Work out the finished part from the listing and answer in its coordinate system (mm). A direction names the side the tool comes from. Round coordinates to 2 decimals unless told otherwise and drop trailing zeros. Order: outer loops, then holes, each group sorted by start corner. A loop starts at its lowest first (then second) coordinate and runs counter-clockwise, first axis right, second up. Notation, with made-up numbers: M 43,63.5 L 63,63.5 A27 cw 63,100.5 Z; hole C 3,3 d3. An arc over 180 degrees is marked long. Return JSON: item names as keys, results as strings.
from build123d import *

# Parameters (mm, degrees)
SKETCH013_W   = 18.2
SKETCH013_H   = 20.2
SKETCH013_W_2 = 7.8
SKETCH013_H_2 = 4.8
PAD013_DEPTH  = 5


with BuildPart() as part:
    # Sketch013 → Pad013 (new body)
    with BuildSketch(Plane(origin=(0, -2.5, 80), x_dir=(1, 0, 0), z_dir=(0, 0, 1))):
        Rectangle(SKETCH013_W, SKETCH013_H)
        with Locations((0, 5)):
            Rectangle(SKETCH013_W_2, SKETCH013_H_2, mode=Mode.SUBTRACT)
        with Locations((0, -5)):
            Rectangle(SKETCH013_W_2, SKETCH013_H_2, mode=Mode.SUBTRACT)
    extrude(amount=PAD013_DEPTH)


solid = part.part
Item 1: Find section B-B (z = 83.45). Determine the outline of the cut face in (x, y).
Output:
{"outline": "M -9.1,-12.6 L 9.1,-12.6 L 9.1,7.6 L -9.1,7.6 Z; hole M -3.9,-9.9 L 3.9,-9.9 L 3.9,-5.1 L -3.9,-5.1 Z; hole M -3.9,0.1 L 3.9,0.1 L 3.9,4.9 L -3.9,4.9 Z"}
Item 2: Find section C-C (x = 1). Determine the outline of the cut face in (y, z).
Output:
{"outline": "M -12.6,80 L -9.9,80 L -9.9,85 L -12.6,85 Z; M -5.1,80 L 0.1,80 L 0.1,85 L -5.1,85 Z; M 4.9,80 L 7.6,80 L 7.6,85 L 4.9,85 Z"}
Item 3: The mould has two halves that part along Y. Classify faces 3 (the flat face through (0, 4.9, 82)), 4 (the flat face through (0, -2, 80)), 5 (the flat face through (0, -12.6, 82)): pulls with the +Y half, pulls with the -Y half, needs draft (parallel to the pull), parting line crosses it, or undercut.
Output:
{"face 3": "undercut", "face 4": "needs draft", "face 5": "pulls with the -Y half"}
Item 4: Consider line 1 along Y through (x, z) = (-3, 83.7); line 2 along X through (y, z) = (0.75, 80.6). Determine where each line is inside the solid, lowest interval first. Write a range as [from, to].
Output:
{"line 1": "y = [-12.6, -9.9], [-5.1, 0.1], [4.9, 7.6]", "line 2": "x = [-9.1, -3.9], [3.9, 9.1]"}
Item 5: Which of the six approach directions +Z, -Z, +X, -X, +Y, -Y give full straight-line access (tool end or side, diameter ignored) to faces 1 (the flat face through (3.9, -8, 82)), 2 (the flat face through (0, -2, 85))?
Output:
{"face 1": "+Z, -Z", "face 2": "+Z, +X, -X, +Y, -Y"}
Item 6: Find section A-A (y = -8.5). Determine the outline of the cut face in (x, z).
Output:
{"outline": "M -9.1,80 L -3.9,80 L -3.9,85 L -9.1,85 Z; M 3.9,80 L 9.1,80 L 9.1,85 L 3.9,85 Z"}
